Here's how the part is built. I have some questions about the finished solid (model axes, mm). A direction names the side the tool comes from. Coordinates: 2 decimals unless noted, no trailing zeros. Order: outer loops, then holes, each group sorted by start corner. A loop starts at its lowest first (then second) coordinate and runs counter-clockwise, first axis right, second up. Notation, with made-up numbers: (-11, -33) - (16, -33) arc R26 ccw to (16, -6) - close; hole circle Ø9 at (34, 34.5). An arc over 180 degrees is marked (long way). Answer as CSV lines item,"result". Start each with the question number.
Q1. For pin 1 Ø1.2 at (x, y) = (-2.5, 0) entering from +Z, with a flat end and sliding along its axis, tell me the tip position at first contact or that it passes through.
Q2. Suppose I cut it at B-B (x = 2.5). Please give me the cut outline in (y, z).
Q3. I need wall thicknesses on line 1 (Z direction, x = 4.5, y = 1.3); line 2 (X direction, y = -1.35, z = -12.5); line 3 (X direction, y = 0.6, z = -5.5). Which ranges of each line are inside material? Lowest first, please.
Q4. Suppose I cut it at D-D (x = -0.5). Please give me the cut outline in (y, z).
Q5. For faces 4 (the face through (3.057, 0.192, 19.616)), 5 (the face through (0, 2, 0)), which set-ups out of +Z, -Z, +X, -X, +Y, -Y let a thin tool reach every point of the face, with its end or its side?
Q6. Suppose I cut it at A-A (y = 0). Please give me the cut outline in (x, z), then the cut area to 4 significant figures.
Q7. Thinking about a two-plate mould opening in X: for faces 1 (the face through (-5.905, -0.022, 19.616)), 2 (the face through (-5.4, 0, 20.25)), 3 (the face through (-8, 0, 0)), which applies, released by +X, released by -X, zero draft, split by the parting line, or undercut?
Q8. Suppose I cut it at C-C (z = -15). Please give me the cut outline in (x, y), then the cut area to 3 significant figures.
Autodesk Inventor part; units mm, degrees
ref_plane "YZ Plane" through (0, 0, 0) normal (1, 0, 0) x (0, 1, 0)
ref_plane "XZ Plane" through (0, 0, 0) normal (0, 1, 0) x (-1, 0, 0)
ref_plane "XY Plane" through (0, 0, 0) normal (0, 0, 1) x (1, 0, 0)
sketch "Sketch1" plane through (0, 0, 0) normal (0, 0, 1) x (1, 0, 0)
  line L0 (-6, 0) -> (6, 0) construction
  line L1 (-6, -2) -> (6, -2)
  line L2 (6, 2) -> (-6, 2)
  arc A0 (-6, 2) -> (-6, -2) centre (-6, 0) ccw
  arc A1 (6, -2) -> (6, 2) centre (6, 0) ccw
  point P0 (0, 0)
  point P1 (0, 0)
  point P2 (-8, 0)
  point P3 (8, 0)
  dimension "d0" = 4
  dimension "d1" = 16
extrude "Extrusion1" add sketch "Sketch1" along normal mid plane 38
sketch "Sketch2" plane through (0, 0, 19) normal (0, 0, 1) x (1, 0, 0)
  circle A0 centre (2.5947, 0) radius 0.5
  circle A1 centre (-5.4053, 0) radius 0.5
  point P0 (0, 0)
  dimension "d4" = 8
  dimension "d5" = 1
extrude "Extrusion2" add sketch "Sketch2" along normal blind 1.25
properties part number "battery"
Here are the results:
1,pin 1,"stops at z = 19"
2,outline,"(-2, -19) - (2, -19) - (2, 19) - (0.49, 19) - (0.49, 20.25) - (-0.49, 20.25) - (-0.49, 19) - (-2, 19) - close"
3,line 1,"z = -19 to 19"
3,line 2,"x = -7.48 to 7.48"
3,line 3,"x = -7.91 to 7.91"
4,outline,"(-2, -19) - (2, -19) - (2, 19) - (-2, 19) - close"
5,face 4,"+Z"
5,face 5,"+Z, -Z, +X, -X, +Y"
6,outline,"(-8, -19) - (8, -19) - (8, 19) - (3.09, 19) - (3.09, 20.25) - (2.09, 20.25) - (2.09, 19) - (-4.91, 19) - (-4.91, 20.25) - (-5.91, 20.25) - (-5.91, 19) - (-8, 19) - close"
6,area,"610.5 mm²"
7,face 1,"undercut"
7,face 2,"zero draft"
7,face 3,"released by -X"
8,outline,"(-6, -2) - (6, -2) arc R2 ccw to (6, 2) - (-6, 2) arc R2 ccw to start"
8,area,"60.6 mm²"
